Study the drawing (mm; zero at the part's minimum x, y, z) and answer. A direction names the side the tool comes from. Round coordinates to 2 decimals unless told otherwise and drop trailing zeros. Loops run counter-clockwise (first coordinate to the right, second up) from the corner with the lowest first, then second, coordinate; pieces in that order, holes last. Notation, with made-up numbers: (-20.75, 47) -> (23.25, 47) arc R32 cw to (23.25, 73) -> close; hole circle Ø11 at (33.25, 59.5). An arc over 180 degrees is marked (long way). Write each question's results on one line, items separated by ' | '. Start each with the question number.
(1) A flat-ended cylindrical pin translates along its axis: pin 1 (5 mm diameter, centred on x = 137.5, y = 165.5, fed in from +Z). Find the tip coordinate at first contact, or state that the pin passes through.
(2) Straight lines are drawn through the part: probe 1 along Y at (x, z) = (88.5, 610.5); probe 2 along X at (y, z) = (121, 471.5); probe 3 along Z at (x, y) = (181, 207). For each, find the intervals that lie inside material, in ascending order.
(3) The part is cut by section B-B (y = 448). Determine the outline of the cut face in (x, z).
(4) For the marked faces 1 and 2, determine the directions among +Z, -Z, +X, -X, +Y, -Y from which every point of the face is accessible in a straight line to the end or side of a thin tool.
(5) Determine the mould class of the marked faces 3, 4, 5 and 6 for opening direction Y: released by +Y, released by -Y, zero draft, split by the parting line, or undercut.
(6) The part is cut by section A-A (x = 300). Determine the outline of the cut face in (y, z), plus the area to 3 significant figures.
(7) The part is cut by section C-C (y = 167.5). Determine the outline of the cut face in (x, z).
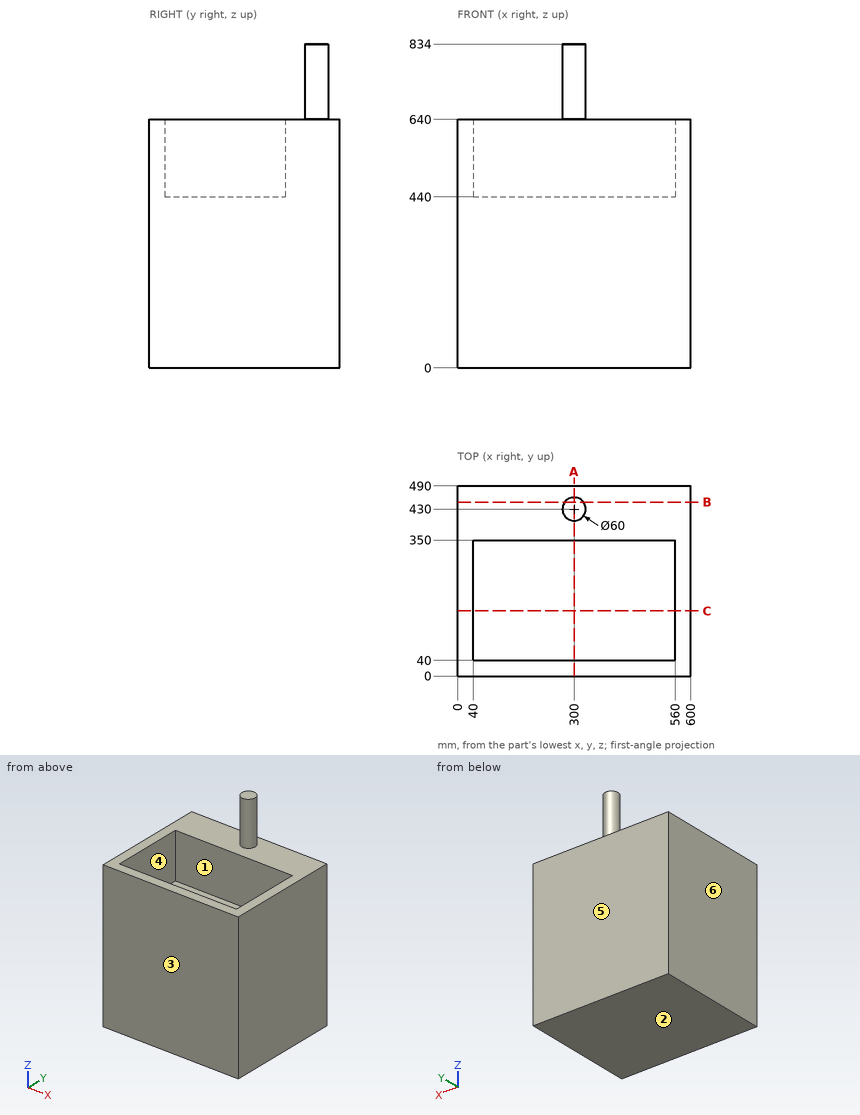
Checked values:
1) pin 1: stops at z = 440
2) probe 1: y = 0 to 40, 350 to 490 | probe 2: x = 0 to 40, 560 to 600 | probe 3: z = 0 to 440
3) outline: (0, 0) -> (600, 0) -> (600, 640) -> (324, 640) -> (324, 834) -> (276, 834) -> (276, 640) -> (0, 640) -> close
4) face 1: +Z | face 2: -Z, +X, -X, +Y, -Y
5) face 3: released by -Y | face 4: undercut | face 5: released by +Y | face 6: zero draft
6) outline: (0, 0) -> (490, 0) -> (490, 640) -> (460, 640) -> (460, 834) -> (400, 834) -> (400, 640) -> (350, 640) -> (350, 440) -> (40, 440) -> (40, 640) -> (0, 640) -> close | area: 263,000 mm2
7) outline: (0, 0) -> (600, 0) -> (600, 640) -> (560, 640) -> (560, 440) -> (40, 440) -> (40, 640) -> (0, 640) -> close
